Could you check a few things on this model? Use its own coordinates, in mm. Face numbers are marked on the shaded views. A direction names the side the tool comes from. Coordinates: 2 decimals unless noted, no trailing zeros. Write each loop counter-clockwise with the first axis right and the second up, starting at its lowest first coordinate (ties: lowest second). Pieces come first, ordered by that corner, then holes.
Item 1: If I drill on probe 1 along X at (y, z) = (36.9, 0) (3 decimals); probe 2 along Y at (x, z) = (2, -4.5); probe 3 along Y at (x, z) = (5.5, 22), over which ranges is the centre line in solid material (lowest first)?
Item 2: Which directions (+Z, -Z, +X, -X, +Y, -Y) give clear straight access to the entire face, cutting with the end or side of a thin tool? Please do the marked faces 5, 6 and 7.
Item 3: For P1, Ø6, axis at y = -7, z = 20, coming from the +X side; P2, Ø2, axis at x = -15, y = 0, coming from the +Z side; P3, Ø1.5, axis at x = 13.5, y = -8, coming from the -Z side, each with a flat end and sliding along its axis, tell me the tip position at first contact or that it passes through.
Item 4: Thinking about a two-plate mould opening in Y: for the marked faces 1, 2, 3 and 4, which applies, +Y half, -Y half, draft (parallel to the pull), parting line (faces both ways), or undercut?
Item 5: I want a section at D-D on z = -15. Please give me the cut outline in (x, y).
Item 6: I want a section at B-B on y = -13. Please give me the cut outline in (x, z), then the cut area to 3 significant figures.
Item 7: I want a section at C-C on y = 9.5. Please give me the cut outline in (x, z), then the cut area to 3 significant figures.
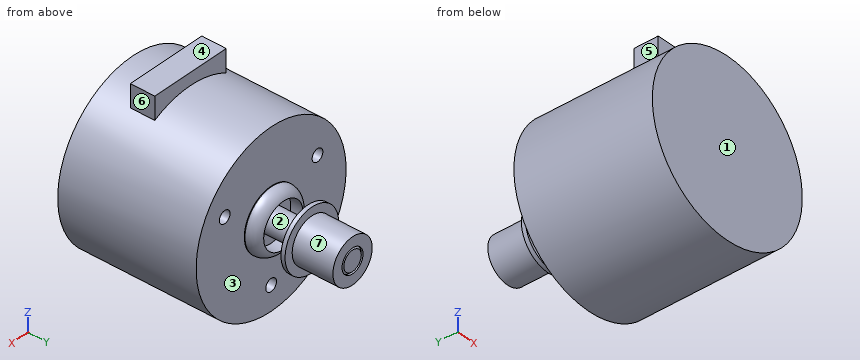
from build123d import *

# Parameters (mm, degrees)
SKETCH1_R           = 21
SKETCH1_R_2         = 1.5
SKETCH1_R_3         = 7.5
SKETCH1_R_4         = 5.5
SKETCH1_R_5         = 2.945
BOSS_EXTRUDE1_DEPTH = 17
CUT_EXTRUDE1_START  = 17
SKETCH1_3_R         = 1.5
CUT_EXTRUDE1_DEPTH  = 10
BOSS_EXTRUDE2_START = 17
SKETCH1_4_R         = 7.5
SKETCH1_4_R_2       = 5.5
BOSS_EXTRUDE2_DEPTH = 3
FILLET1_R           = 3
BOSS_EXTRUDE3_START = 17
SKETCH1_5_R         = 2.945
BOSS_EXTRUDE3_DEPTH = 20
BOSS_EXTRUDE4_START = -2.8
BOSS_EXTRUDE4_DEPTH = 6
CHAMFER1_SIZE       = 0.5
BOSS_EXTRUDE6_START = 27
SKETCH1_10_R        = 5.5
SKETCH1_10_R_2      = 2.945
BOSS_EXTRUDE6_DEPTH = 10
BOSS_EXTRUDE7_START = 26
SKETCH1_12_R        = 7.5
SKETCH1_12_R_2      = 5.5
SKETCH1_12_R_3      = 2.945
BOSS_EXTRUDE7_DEPTH = 1


with BuildPart() as part:
    # Sketch1 → Boss-Extrude1 (new, symmetric)
    # profile 1 of 7: a face of its own
    with BuildSketch(Plane(origin=(0, 0, 0), x_dir=(1, 0, 0), z_dir=(0, 1, 0))):
        with Locations(Location((0, 0, 0), (0, 0, 270))):
            Circle(SKETCH1_R)
        with Locations((12.990381057, -7.5)):
            Circle(SKETCH1_R_2, mode=Mode.SUBTRACT)
        with Locations((-12.990381057, -7.5)):
            Circle(SKETCH1_R_2, mode=Mode.SUBTRACT)
        with Locations((0, 15)):
            Circle(SKETCH1_R_2, mode=Mode.SUBTRACT)
        Circle(SKETCH1_R_3, mode=Mode.SUBTRACT)
    # profile 2 of 7: a face of its own
    with BuildSketch(Plane(origin=(0, 0, 0), x_dir=(1, 0, 0), z_dir=(0, 1, 0))):
        Circle(SKETCH1_R_3)
        Circle(SKETCH1_R_4, mode=Mode.SUBTRACT)
    # profile 3 of 7: a face of its own
    with BuildSketch(Plane(origin=(0, 0, 0), x_dir=(1, 0, 0), z_dir=(0, 1, 0))):
        Circle(SKETCH1_R_4)
        Circle(SKETCH1_R_5, mode=Mode.SUBTRACT)
    # profile 4 of 7: a face of its own
    with BuildSketch(Plane(origin=(0, 0, 0), x_dir=(1, 0, 0), z_dir=(0, 1, 0))):
        Circle(SKETCH1_R_5)
    # profile 5 of 7: a face of its own
    with BuildSketch(Plane(origin=(0, 0, 0), x_dir=(1, 0, 0), z_dir=(0, 1, 0))):
        with Locations((-12.990381057, -7.5)):
            Circle(SKETCH1_R_2)
    # profile 6 of 7: a face of its own
    with BuildSketch(Plane(origin=(0, 0, 0), x_dir=(1, 0, 0), z_dir=(0, 1, 0))):
        with Locations((12.990381057, -7.5)):
            Circle(SKETCH1_R_2)
    # profile 7 of 7: a face of its own
    with BuildSketch(Plane(origin=(0, 0, 0), x_dir=(1, 0, 0), z_dir=(0, 1, 0))):
        with Locations((0, 15)):
            Circle(SKETCH1_R_2)
    extrude(amount=BOSS_EXTRUDE1_DEPTH, both=True)

    # Sketch1<3> → Cut-Extrude1 (cut)
    with BuildSketch(Plane(origin=(0, 0, 0), x_dir=(1, 0, 0), z_dir=(0, 1, 0)).offset(CUT_EXTRUDE1_START)):
        with Locations(Location((-12.990381057, -7.5, 0), (0, 0, 270))):
            Circle(SKETCH1_3_R)
        with Locations(Location((12.990381057, -7.5, 0), (0, 0, 270))):
            Circle(SKETCH1_3_R)
        with Locations(Location((0, 15, 0), (0, 0, 270))):
            Circle(SKETCH1_3_R)
    extrude(amount=-CUT_EXTRUDE1_DEPTH, mode=Mode.SUBTRACT)

    # Sketch1<4> → Boss-Extrude2 (add)
    with BuildSketch(Plane(origin=(0, 0, 0), x_dir=(1, 0, 0), z_dir=(0, 1, 0)).offset(BOSS_EXTRUDE2_START)):
        with Locations(Location((0, 0, 0), (0, 0, 270))):
            Circle(SKETCH1_4_R)
        with Locations(Location((0, 0, 0), (0, 0, 270))):
            Circle(SKETCH1_4_R_2, mode=Mode.SUBTRACT)
    extrude(amount=BOSS_EXTRUDE2_DEPTH)

    # Fillet1
    # the kernel refuses this fillet: 3 mm, written as the material it takes off along each edge
    with BuildSketch(Plane(origin=(0, 20, 0), x_dir=(0, 0, 1), z_dir=(-1, 0, 0))) as fillet1_piece_1:
        with BuildLine():
            CenterArc((4.5, -2.828427125), FILLET1_R, 0, 70.528779366)
            Line((5.5, 0), (5.52, 0.056568542))
            ThreePointArc((5.52, 0.056568542), (6.5, 0.06), (7.5, 0.06))
            Line((7.5, 0.06), (7.56, 0))
            Line((7.56, 0), (7.56, -2.828427125))
            Line((7.56, -2.828427125), (7.5, -2.828427125))
        make_face()
    revolve(axis=Axis((0, 20, 0), (0, 1, 0)), mode=Mode.SUBTRACT)

    # Sketch1<5> → Boss-Extrude3 (add)
    with BuildSketch(Plane(origin=(0, 0, 0), x_dir=(1, 0, 0), z_dir=(0, 1, 0)).offset(BOSS_EXTRUDE3_START)):
        with Locations(Location((0, 0, 0), (0, 0, 270))):
            Circle(SKETCH1_5_R)
    extrude(amount=BOSS_EXTRUDE3_DEPTH)

    # Sketch1<8> → Boss-Extrude4 (add)
    with BuildSketch(Plane(origin=(0, 0, 0), x_dir=(1, 0, 0), z_dir=(0, 1, 0)).offset(BOSS_EXTRUDE4_START)):
        with BuildLine():
            ThreePointArc((10, -18.466185313), (0, -21), (-10, -18.466185313))
            Line((-10, -18.466185313), (-10, -24))
            Line((-10, -24), (10, -24))
            Line((10, -24), (10, -18.466185313))
        make_face()
    extrude(amount=-BOSS_EXTRUDE4_DEPTH)

    # Chamfer1
    chamfer1_edges = [part.edges().sort_by_distance(p)[0] for p in [
        (0, 37, -2.945),
    ]]
    chamfer(chamfer1_edges, length=CHAMFER1_SIZE)

    # Sketch1<10> → Boss-Extrude6 (add)
    with BuildSketch(Plane(origin=(0, 0, 0), x_dir=(1, 0, 0), z_dir=(0, 1, 0)).offset(BOSS_EXTRUDE6_START)):
        with Locations(Location((0, 0, 0), (0, 0, 270))):
            Circle(SKETCH1_10_R)
        with Locations(Location((0, 0, 0), (0, 0, 270))):
            Circle(SKETCH1_10_R_2, mode=Mode.SUBTRACT)
    extrude(amount=BOSS_EXTRUDE6_DEPTH)

    # Sketch1<12> → Boss-Extrude7 (add)
    # profile 1 of 2: a face of its own
    with BuildSketch(Plane(origin=(0, 0, 0), x_dir=(1, 0, 0), z_dir=(0, 1, 0)).offset(BOSS_EXTRUDE7_START)):
        with Locations(Location((0, 0, 0), (0, 0, 270))):
            Circle(SKETCH1_12_R)
        with Locations(Location((0, 0, 0), (0, 0, 270))):
            Circle(SKETCH1_12_R_2, mode=Mode.SUBTRACT)
    # profile 2 of 2: a face of its own
    with BuildSketch(Plane(origin=(0, 0, 0), x_dir=(1, 0, 0), z_dir=(0, 1, 0)).offset(BOSS_EXTRUDE7_START)):
        with Locations(Location((0, 0, 0), (0, 0, 270))):
            Circle(SKETCH1_12_R_2)
        with Locations(Location((0, 0, 0), (0, 0, 270))):
            Circle(SKETCH1_12_R_3, mode=Mode.SUBTRACT)
    extrude(amount=BOSS_EXTRUDE7_DEPTH)


solid = part.part
Response values:
1. probe 1: x = -5.5 to -2.945, -2.545 to 2.545, 2.945 to 5.5
1. probe 2: y = -17 to 17, 26 to 37
1. probe 3: y = -8.8 to -2.8
2. face 5: +Z, -X, +Y, -Y
2. face 6: +Z, +X, +Y, -Y
2. face 7: +Y
3. P1: stops at x = 12.33
3. P2: stops at z = 15.65
3. P3: stops at z = -16.69
4. face 1: -Y half
4. face 2: undercut
4. face 3: +Y half
4. face 4: draft
5. outline: (-14.7, -17) - (14.7, -17) - (14.7, 17) - (1.5, 17) - (1.5, 7) - (-1.5, 7) - (-1.5, 17) - (-14.7, 17) - close
6. outline: circle Ø42 at (0, 0)
6. area: 1,390 mm2
7. outline: circle Ø42 at (0, 0); hole circle Ø3 at (-12.99, 7.5); hole circle Ø3 at (0, -15); hole circle Ø3 at (12.99, 7.5)
7. area: 1,360 mm2
